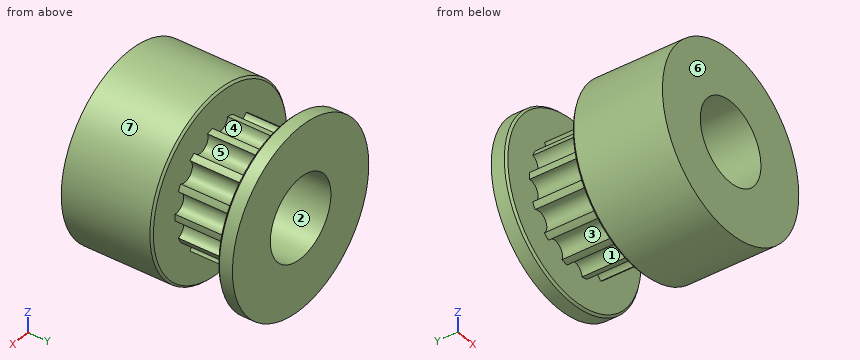
from build123d import *

# Parameters (mm, degrees)
SKETCH_2_R          = 9
EXTRUDE_1_DEPTH     = 9
EXTRUDE_2_DEPTH     = 6.5
SKETCH_4_R          = 9
EXTRUDE_3_DEPTH     = 1.5
SKETCH_5_R          = 4
CUT_EXTRUDE_1_DEPTH = 22.236760582
CHAMFER_1_SIZE      = 0.2


with BuildPart() as part:
    # 草图2 → 凸台-拉伸1 (new body)
    with BuildSketch(Plane(origin=(0, 0, 0), x_dir=(1, 0, 0), z_dir=(0, 1, 0))):
        with Locations(Location((0, 0, 0), (0, 0, 270))):
            Circle(SKETCH_2_R)
    extrude(amount=EXTRUDE_1_DEPTH)

    # 草图3 → 凸台-拉伸2 (add)
    with BuildSketch(Plane(origin=(0, 9, 0), x_dir=(1, 0, 0), z_dir=(0, 1, 0))):
        with BuildLine():
            ThreePointArc((-3.444184526, 4.855302323), (-3.711538364, 4.654121901), (-3.967166599, 4.438238037))
            ThreePointArc((-3.967166599, 4.438238037), (-3.872290418, 3.088048563), (-5.20973976, 2.880100577))
            ThreePointArc((-5.20973976, 2.880100577), (-5.363328331, 2.582842797), (-5.499972914, 2.277425222))
            ThreePointArc((-5.499972914, 2.277425222), (-4.828667171, 1.102111772), (-5.943442141, 0.334459589))
            ThreePointArc((-5.943442141, 0.334459589), (-5.952845345, 0), (-5.943442141, -0.334459589))
            ThreePointArc((-5.943442141, -0.334459589), (-4.828667171, -1.102111772), (-5.499972914, -2.277425222))
            ThreePointArc((-5.499972914, -2.277425222), (-5.363328331, -2.582842797), (-5.20973976, -2.880100577))
            ThreePointArc((-5.20973976, -2.880100577), (-3.872290418, -3.088048563), (-3.967166599, -4.438238037))
            ThreePointArc((-3.967166599, -4.438238037), (-3.711538364, -4.654121901), (-3.444184526, -4.855302323))
            ThreePointArc((-3.444184526, -4.855302323), (-2.148959057, -4.462359463), (-1.648614285, -5.720003377))
            ThreePointArc((-1.648614285, -5.720003377), (-1.324632706, -5.803595083), (-0.996466307, -5.868851898))
            ThreePointArc((-0.996466307, -5.868851898), (0, -4.952845345), (0.996466307, -5.868851898))
            ThreePointArc((0.996466307, -5.868851898), (1.324632706, -5.803595083), (1.648614285, -5.720003377))
            ThreePointArc((1.648614285, -5.720003377), (2.148959057, -4.462359463), (3.444184526, -4.855302323))
            ThreePointArc((3.444184526, -4.855302323), (3.711538364, -4.654121901), (3.967166599, -4.438238037))
            ThreePointArc((3.967166599, -4.438238037), (3.872290418, -3.088048563), (5.20973976, -2.880100577))
            ThreePointArc((5.20973976, -2.880100577), (5.363328331, -2.582842797), (5.499972914, -2.277425222))
            ThreePointArc((5.499972914, -2.277425222), (4.828667171, -1.102111772), (5.943442141, -0.334459589))
            ThreePointArc((5.943442141, -0.334459589), (5.952845345, 0), (5.943442141, 0.334459589))
            ThreePointArc((5.943442141, 0.334459589), (4.828667171, 1.102111772), (5.499972914, 2.277425222))
            ThreePointArc((5.499972914, 2.277425222), (5.363328331, 2.582842797), (5.20973976, 2.880100577))
            ThreePointArc((5.20973976, 2.880100577), (3.872290418, 3.088048563), (3.967166599, 4.438238037))
            ThreePointArc((3.967166599, 4.438238037), (3.711538364, 4.654121901), (3.444184526, 4.855302323))
            ThreePointArc((3.444184526, 4.855302323), (2.148959057, 4.462359463), (1.648614285, 5.720003377))
            ThreePointArc((1.648614285, 5.720003377), (1.324632706, 5.803595083), (0.996466307, 5.868851898))
            ThreePointArc((0.996466307, 5.868851898), (0, 4.952845345), (-0.996466307, 5.868851898))
            ThreePointArc((-0.996466307, 5.868851898), (-1.324632706, 5.803595083), (-1.648614285, 5.720003377))
            ThreePointArc((-1.648614285, 5.720003377), (-2.148959057, 4.462359463), (-3.444184526, 4.855302323))
        make_face()
    extrude(amount=EXTRUDE_2_DEPTH)

    # 草图4 → 凸台-拉伸3 (add)
    with BuildSketch(Plane(origin=(0, 15.5, 0), x_dir=(1, 0, 0), z_dir=(0, 1, 0))):
        with Locations(Location((0, 0, 0), (0, 0, 270))):
            Circle(SKETCH_4_R)
    extrude(amount=EXTRUDE_3_DEPTH)

    # 草图5 → 切除-拉伸1 (cut, through all)
    with BuildSketch(Plane(origin=(0, 17, 0), x_dir=(1, 0, 0), z_dir=(0, 1, 0))):
        with Locations(Location((0, 0, 0), (0, 0, 270))):
            Circle(SKETCH_5_R)
    extrude(amount=-CUT_EXTRUDE_1_DEPTH, mode=Mode.SUBTRACT)

    # 倒角1
    chamfer_1_edges = [part.edges().sort_by_distance(p)[0] for p in [
        (0, 9, -9),
        (0, 15.5, -9),
    ]]
    chamfer(chamfer_1_edges, length=CHAMFER_1_SIZE)


solid = part.part
The model under review builds one solid part; all positions refer to its coordinate system, in mm. Face numbers are marked on the shaded views. A direction names the side the tool comes from. Round coordinates to 2 decimals unless told otherwise and drop trailing zeros. Loops run counter-clockwise (first coordinate to the right, second up) from the corner with the lowest first, then second, coordinate; pieces in that order, holes last. Notation, with made-up numbers: (89.25, -26.5) -> (96.25, -26.5) arc R5 cw to (96.25, -19.5) -> close; hole circle Ø9 at (48.25, 57.25). An arc over 180 degrees is marked (long way). One line per question, with ' | ' between items. Start each with the question number.
Item 1: Add section D-D, the plane y = 4. Write out the cut boundary in (x, z), then the cut area to 3 significant figures.
Item 2: Machinability: for the marked faces 1, 2 and 3, which of the approach directions +Z, -Z, +X, -X, +Y, -Y give a long, thin tool a straight path to every point of the face, cutting with its end or side? Answer none if there is none.
Item 3: Wall thickness on line 1 along X through (y, z) = (5.5, 0); line 2 along Y through (x, z) = (5, -4.5); line 3 along Y through (x, z) = (-5.5, -7): over which ranges is each line inside the solid? List them lowest first. Write a range as [from, to].
Item 4: Draft analysis for pull direction X (two halves, no side actions). For the marked faces 4, 5, 6 and 7, state which applies: +X half, -X half, draft (parallel to the pull), parting line (faces both ways), or undercut.
Item 5: Add section B-B, the plane z = 0. Write out the cut boundary in (x, y), then the cut area to 3 significant figures.
Item 6: Add section C-C, the plane x = 0. Write out the cut boundary in (y, z).
Item 7: For pin 1 (2 mm diameter, centred on x = -4, y = 6, fed in from -Z); pin 2 (5 mm diameter, centred on x = 0, z = 0, fed in from -Y); pin 3 (1.5 mm diameter, centred on x = -5, z = -2, fed in from -Y); pin 4 (1 mm diameter, centred on x = -1, y = 7.5, fed in from -Z), all flat-tipped, find the tip position at first contact; note any pin that passes through.
Return value:
1) outline: circle Ø18 at (0, 0); hole circle Ø8 at (0, 0) | area: 204 mm2
2) face 1: -Z | face 2: +Y, -Y | face 3: none
3) line 1: x = [-9, -4], [4, 9] | line 2: y = [0, 9], [15.5, 17] | line 3: y = [0, 8.9], [15.6, 17]
4) face 4: undercut | face 5: undercut | face 6: draft | face 7: parting line
5) outline: (-9, 0) -> (-4, 0) -> (-4, 17) -> (-9, 17) -> (-9, 15.7) -> (-8.8, 15.5) -> (-5.95, 15.5) -> (-5.95, 9) -> (-8.8, 9) -> (-9, 8.8) -> close; (4, 0) -> (9, 0) -> (9, 8.8) -> (8.8, 9) -> (5.95, 9) -> (5.95, 15.5) -> (8.8, 15.5) -> (9, 15.7) -> (9, 17) -> (4, 17) -> close | area: 130 mm2
6) outline: (0, -9) -> (8.8, -9) -> (9, -8.8) -> (9, -4.95) -> (15.5, -4.95) -> (15.5, -8.8) -> (15.7, -9) -> (17, -9) -> (17, -4) -> (0, -4) -> close; (0, 4) -> (17, 4) -> (17, 9) -> (15.7, 9) -> (15.5, 8.8) -> (15.5, 4.95) -> (9, 4.95) -> (9, 8.8) -> (8.8, 9) -> (0, 9) -> close
7) pin 1: stops at z = -8.49 | pin 2: passes through | pin 3: stops at y = 0 | pin 4: stops at z = -8.99
